Read the model definition and answer for the solid it produces. Units are mm, in the model's axes. A direction names the side the tool comes from. Coordinates: 2 decimals unless noted, no trailing zeros. Order: outer loops, then holes, each group sorted by start corner. A loop starts at its lowest first (then second) coordinate and runs counter-clockwise, first axis right, second up. Notation, with made-up numbers: (-17, 20) -> (25, 20) arc R32 ccw to (25, 57) -> close; hole circle Ø9 at (70, 82). An arc over 180 degrees is marked (long way). Answer in a Markdown table with one row per item.
from build123d import *

# Parameters (mm, degrees)
SKETCH1_R           = 2.4
BOSS_EXTRUDE1_DEPTH = 60
SKETCH6_R           = 1.25
BOSS_EXTRUDE2_DEPTH = 2.5
SKETCH7_R           = 1.3
CUT_EXTRUDE1_DEPTH  = 2.5
JOIN2_START         = 2
JOIN2_OUTLINE_R     = 2.4
JOIN2_DEPTH         = 10


# Read off the part's stored shape, not the designer's step: Join2
with BuildPart() as part:
    # Sketch1 → Boss-Extrude1 (new body)
    with BuildSketch(Plane.XY):
        Circle(SKETCH1_R)
    extrude(amount=BOSS_EXTRUDE1_DEPTH)

    # Sketch6 → Boss-Extrude2 (add)
    with BuildSketch(Plane(origin=(0, 0, 0), x_dir=(-1, 0, 0), z_dir=(0, 0, -1))):
        Circle(SKETCH6_R)
    extrude(amount=BOSS_EXTRUDE2_DEPTH)

    # Sketch7 → Cut-Extrude1 (cut)
    with BuildSketch(Plane.XY.offset(60)):
        Circle(SKETCH7_R)
    extrude(amount=-CUT_EXTRUDE1_DEPTH, mode=Mode.SUBTRACT)

    # Join2 outline → Join2 (add)
    with BuildSketch(Plane.XY.offset(JOIN2_START)):
        with BuildLine():
            ThreePointArc((2.986969532, 3.160983077), (3.378378938, 3.767383023), (3.534131338, 4.472126528))
            ThreePointArc((3.534131338, 4.472126528), (3.42105158, 4.559211126), (3.305826871, 4.643437164))
            ThreePointArc((3.305826871, 4.643437164), (2.672723858, 4.296878666), (2.199922956, 3.751551677))
            ThreePointArc((2.199922956, 3.751551677), (1.926567958, 3.89899178), (1.643387346, 4.026546788))
            ThreePointArc((1.643387346, 4.026546788), (1.78930882, 4.733391284), (1.679960889, 5.446809287))
            ThreePointArc((1.679960889, 5.446809287), (1.54305857, 5.487164136), (1.405188775, 5.524078612))
            ThreePointArc((1.405188775, 5.524078612), (0.940029166, 4.972219249), (0.696150284, 4.29292159))
            ThreePointArc((0.696150284, 4.29292159), (0.387992831, 4.331658177), (0.077856591, 4.348303043))
            ThreePointArc((0.077856591, 4.348303043), (-0.04141737, 5.060128822), (-0.401097586, 5.68587027))
            ThreePointArc((-0.401097586, 5.68587027), (-0.54333305, 5.674045223), (-0.685227852, 5.658662633))
            ThreePointArc((-0.685227852, 5.658662633), (-0.919621674, 4.976034071), (-0.90164134, 4.254508655))
            ThreePointArc((-0.90164134, 4.254508655), (-1.202982876, 4.179310134), (-1.498189127, 4.082796877))
            ThreePointArc((-1.498189127, 4.082796877), (-1.866549914, 4.703467924), (-2.427985611, 5.157022966))
            ThreePointArc((-2.427985611, 5.157022966), (-2.556344531, 5.094615063), (-2.683100661, 5.02901291))
            ThreePointArc((-2.683100661, 5.02901291), (-2.655072511, 4.307807918), (-2.377661306, 3.64150075))
            ThreePointArc((-2.377661306, 3.64150075), (-2.631489081, 3.4625231), (-2.871896102, 3.26588637))
            ThreePointArc((-2.871896102, 3.26588637), (-3.439594549, 3.71157762), (-4.126960724, 3.931691135))
            ThreePointArc((-4.126960724, 3.931691135), (-4.224107518, 3.827128908), (-4.318605858, 3.720167126))
            ThreePointArc((-4.318605858, 3.720167126), (-4.031941094, 3.057788434), (-3.532564937, 2.536687991))
            ThreePointArc((-3.532564937, 2.536687991), (-3.704598104, 2.278103134), (-3.857737594, 2.007899811))
            ThreePointArc((-3.857737594, 2.007899811), (-4.548102881, 2.218418192), (-5.268566924, 2.17536263))
            ThreePointArc((-5.268566924, 2.17536263), (-5.321381378, 2.042767787), (-5.370859403, 1.908892158))
            ThreePointArc((-5.370859403, 1.908892158), (-4.864273689, 1.39479768), (-4.210376099, 1.089281462))
            ThreePointArc((-4.210376099, 1.089281462), (-4.277380625, 0.786012716), (-4.322570249, 0.478735257))
            ThreePointArc((-4.322570249, 0.478735257), (-5.042364718, 0.425649095), (-5.698623966, 0.125239347))
            ThreePointArc((-5.698623966, 0.125239347), (-5.699973196, -0.017480443), (-5.697748625, -0.160189273))
            ThreePointArc((-5.697748625, -0.160189273), (-5.039659169, -0.45656823), (-4.319552638, -0.505238564))
            ThreePointArc((-4.319552638, -0.505238564), (-4.272479191, -0.812233074), (-4.203615838, -1.115085146))
            ThreePointArc((-4.203615838, -1.115085146), (-4.855627257, -1.424606272), (-5.359050265, -1.941798203))
            ThreePointArc((-5.359050265, -1.941798203), (-5.308752049, -2.075367842), (-5.255125323, -2.207636255))
            ThreePointArc((-5.255125323, -2.207636255), (-4.534410753, -2.246272071), (-3.845349658, -2.031523322))
            ThreePointArc((-3.845349658, -2.031523322), (-3.690555767, -2.300782287), (-3.516939816, -2.558307122))
            ThreePointArc((-3.516939816, -2.558307122), (-4.013110431, -3.082460667), (-4.295707129, -3.746585146))
            ThreePointArc((-4.295707129, -3.746585146), (-4.200554521, -3.852965314), (-4.102768227, -3.956929729))
            ThreePointArc((-4.102768227, -3.956929729), (-3.416765039, -3.732604421), (-2.851810899, -3.283439599))
            ThreePointArc((-2.851810899, -3.283439599), (-2.610202337, -3.478598103), (-2.355281584, -3.656015544))
            ThreePointArc((-2.355281584, -3.656015544), (-2.628600803, -4.324011669), (-2.652204943, -5.045375005))
            ThreePointArc((-2.652204943, -5.045375005), (-2.52504883, -5.110198471), (-2.396309547, -5.171817916))
            ThreePointArc((-2.396309547, -5.171817916), (-1.837666272, -4.714827862), (-1.473119275, -4.091909163))
            ThreePointArc((-1.473119275, -4.091909163), (-1.177326617, -4.186609969), (-0.875529522, -4.259958809))
            ThreePointArc((-0.875529522, -4.259958809), (-0.889084071, -4.981580935), (-0.650507783, -5.662759012))
            ThreePointArc((-0.650507783, -5.662759012), (-0.508521301, -5.677271007), (-0.366215984, -5.688223436))
            ThreePointArc((-0.366215984, -5.688223436), (-0.010380493, -5.060287674), (0.104525269, -4.347743722))
            ThreePointArc((0.104525269, -4.347743722), (0.414553585, -4.329196961), (0.722467652, -4.288571031))
            ThreePointArc((0.722467652, -4.288571031), (0.970508391, -4.966360091), (1.439044058, -5.515356036))
            ThreePointArc((1.439044058, -5.515356036), (1.576684846, -5.477596635), (1.713337076, -5.436402861))
            ThreePointArc((1.713337076, -5.436402861), (1.818307229, -4.722327595), (1.668053097, -4.016391398))
            ThreePointArc((1.668053097, -4.016391398), (1.950446029, -3.887101914), (2.222891567, -3.737987972))
            ThreePointArc((2.222891567, -3.737987972), (2.699028318, -4.280404798), (3.334245025, -4.623073665))
            ThreePointArc((3.334245025, -4.623073665), (3.448950969, -4.538142485), (3.56149447, -4.450365955))
            ThreePointArc((3.56149447, -4.450365955), (3.401422484, -3.746591007), (3.006301111, -3.142603161))
            ThreePointArc((3.006301111, -3.142603161), (3.222919929, -2.920032214), (3.423101659, -2.682568924))
            ThreePointArc((3.423101659, -2.682568924), (4.063029514, -3.016357118), (4.779137726, -3.106419579))
            ThreePointArc((4.779137726, -3.106419579), (4.855417152, -2.985787046), (4.928652302, -2.863282467))
            ThreePointArc((4.928652302, -2.863282467), (4.525156785, -2.264856544), (3.938531501, -1.844388954))
            ThreePointArc((3.938531501, -1.844388954), (4.060120634, -1.558595984), (4.161002903, -1.264854079))
            ThreePointArc((4.161002903, -1.264854079), (4.87829606, -1.344933695), (5.578581394, -1.170226315))
            ThreePointArc((5.578581394, -1.170226315), (5.606132343, -1.030184521), (5.630168329, -0.889496816))
            ThreePointArc((5.630168329, -0.889496816), (5.037743587, -0.477240654), (4.338841388, -0.297079798))
            ThreePointArc((4.338841388, -0.297079798), (4.348979549, 0.013337271), (4.336937648, 0.323686319))
            ThreePointArc((4.336937648, 0.323686319), (5.034721691, 0.508130476), (5.624606733, 0.924012497))
            ThreePointArc((5.624606733, 0.924012497), (5.599708298, 1.064550132), (5.571298926, 1.204420309))
            ThreePointArc((5.571298926, 1.204420309), (4.869955203, 1.374829231), (4.153166704, 1.290351631))
            ThreePointArc((4.153166704, 1.290351631), (4.050484678, 1.583469253), (3.927144933, 1.868511086))
            ThreePointArc((3.927144933, 1.868511086), (4.511180261, 2.29256881), (4.910997766, 2.893458301))
            ThreePointArc((4.910997766, 2.893458301), (4.837012617, 3.01551139), (4.759994731, 3.135673797))
            ThreePointArc((4.759994731, 3.135673797), (4.044452383, 3.04122081), (3.406583842, 2.703513922))
            ThreePointArc((3.406583842, 2.703513922), (3.204949406, 2.939744939), (2.986969532, 3.160983077))
        make_face()
        Circle(JOIN2_OUTLINE_R, mode=Mode.SUBTRACT)
    extrude(amount=JOIN2_DEPTH)


solid = part.part
Q1. The part is cut by section A-A (z = 35). Write down the section's boundary in (x, y), then the cut area to 3 significant figures.
Outcome:
| item | result |
|---|---|
| outline | circle Ø4.8 at (0, 0) |
| area | 18.1 mm² |
Q2. Given pin 1 (1 mm diameter, centred on x = -4, y = 1.5, fed in from +Z); pin 2 (1.3 mm diameter, centred on x = 0.5, y = 0, fed in from +Z), each flat-ended and moving along its own axis, determine where each tip first touches the part or whether it passes through.
Outcome:
| item | result |
|---|---|
| pin 1 | z = 12 |
| pin 2 | z = 57.5 |
Q3. For a pull along Y with two mould halves and no side action, classify faces 1 (the face through (-2.626, -4.314, 6.93)), 2 (the face through (-3.431, 3.707, 6.93)), 3 (the face through (0.27, -1.22, -1.23)) as pulls with the +Y half, pulls with the -Y half, needs draft (parallel to the pull), parting line crosses it, or undercut.
Outcome:
| item | result |
|---|---|
| face 1 | undercut |
| face 2 | pulls with the +Y half |
| face 3 | parting line crosses it |
Q4. Consider line 1 (Y direction, x = 0, z = 58.8); line 2 (Y direction, x = 3.25, z = 4); line 3 (Z direction, x = 1.5, y = -4.75). Determine where each line is inside the solid, lowest interval first.
Outcome:
| item | result |
|---|---|
| line 1 | -2.4 to -1.3, 1.3 to 2.4 |
| line 2 | -4.59 to -3.46, -2.89 to 2.89, 3.51 to 4.62 |
| line 3 | 2 to 12 |
Q5. For faces 4 (the face through (1.79, 4.72, 6.93)), 5 (the face through (1.29, 2.024, 35.664)), 6 (the face through (-4.04, 3.07, 6.93)), determine the directions among +Z, -Z, +X, -X, +Y, -Y from which every point of the face is accessible in a straight line to the end or side of a thin tool.
Outcome:
| item | result |
|---|---|
| face 4 | +Z, -Z |
| face 5 | +Z |
| face 6 | +Z, -Z, -X |
